Input: part model. Units: mm. Frame: model coordinates. Face numbers are marked on the shaded views. Coordinates: 2 decimals unless noted, no trailing zeros. Loops run counter-clockwise (first coordinate to the right, second up) from the corner with the lowest first, then second, coordinate; pieces in that order, holes last. Notation, with made-up numbers: (85, -27) -> (137, -27) arc R19 ccw to (137, 2) -> close; hole circle Ø1 at (69.5, 51.25). An arc over 180 degrees is marked (long way). Put each result on its own line as item: value. Start each with the question number.
1) Cut plane C-C (y = 18.5). Return the cut outline in (x, z), plus the area to 3 significant figures.
2) Pull-direction query (X, two-part tool) for the marked faces 1, 2, 3 and 4; classes: pulls with the +X half, pulls with the -X half, needs draft (parallel to the pull), parting line crosses it, or undercut.
3) Cut plane A-A (z = 0). Return the cut outline in (x, y), plus the area to 3 significant figures.
4) Material intervals for L1, parallel to X at y = 16, z = -14; L2, parallel to X at y = 15.75, z = 0; L3, parallel to X at y = 3.5, z = 11, sorted ascending.
5) Cut plane B-B (x = 0). Return the cut outline in (y, z).
6) Contact query for flat-ended pins moving along their axis: P1, Ø1.5, axis at x = -18.5, y = 4, coming from the -Z side; P2, Ø6, axis at x = -8, y = 13.5, coming from the -Z side; P3, Ø1.5, axis at x = 1.5, y = 8, coming from the -Z side. Output: stop coordinate, or through.
7) Cut plane D-D (x = -14). Return the cut outline in (y, z), plus the area to 3 significant figures.
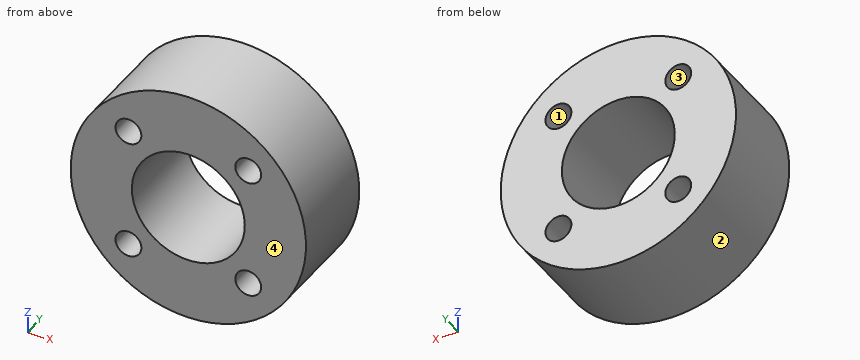
from build123d import *

# Parameters (mm, degrees)
SKETCH_1_R          = 25
EXTRUDE_1_DEPTH     = 20
SKETCH_2_R          = 12
CUT_EXTRUDE_1_DEPTH = 41.620192023
HOLE_WIZARD_M5_1_D  = 5.5


with BuildPart() as part:
    # ｽｹｯﾁ1 → ﾎﾞｽ - 押し出し1 (new body)
    with BuildSketch(Plane(origin=(0, 0, 0), x_dir=(1, 0, 0), z_dir=(0, 1, 0))):
        with Locations(Location((0, 0, 0), (0, 0, 270))):
            Circle(SKETCH_1_R)
    extrude(amount=EXTRUDE_1_DEPTH)

    # ｽｹｯﾁ2 → ｶｯﾄ - 押し出し1 (cut, through all)
    with BuildSketch(Plane(origin=(0, 20, 0), x_dir=(1, 0, 0), z_dir=(0, 1, 0))):
        with Locations(Location((0, 0, 0), (0, 0, 270))):
            Circle(SKETCH_2_R)
    extrude(amount=-CUT_EXTRUDE_1_DEPTH, mode=Mode.SUBTRACT)

    # M5 すきま穴1 (through all)
    with Locations(Plane.XZ):
        with Locations((-12.727922061, 12.727922061), (12.727922061, -12.727922061), (-12.727922061, -12.727922061), (12.727922061, 12.727922061)):
            Hole(HOLE_WIZARD_M5_1_D / 2)


solid = part.part
Results found:
1. outline: circle Ø50 at (0, 0); hole circle Ø5.5 at (-12.73, -12.73); hole circle Ø5.5 at (-12.73, 12.73); hole circle Ø24 at (0, 0); hole circle Ø5.5 at (12.73, -12.73); hole circle Ø5.5 at (12.73, 12.73)
1. area: 1,420 mm2
2. face 1: undercut
2. face 2: parting line crosses it
2. face 3: undercut
2. face 4: needs draft
3. outline: (-25, 0) -> (-12, 0) -> (-12, 20) -> (-25, 20) -> close; (12, 0) -> (25, 0) -> (25, 20) -> (12, 20) -> close
3. area: 520 mm2
4. L1: x = -20.71 to -15.17, -10.29 to 10.29, 15.17 to 20.71
4. L2: x = -25 to -12, 12 to 25
4. L3: x = -22.45 to -14.87, -10.59 to -4.8, 4.8 to 10.59, 14.87 to 22.45
5. outline: (0, -25) -> (20, -25) -> (20, -12) -> (0, -12) -> close; (0, 12) -> (20, 12) -> (20, 25) -> (0, 25) -> close
6. P1: stops at z = -17.61
6. P2: stops at z = -24.49
6. P3: stops at z = -24.99
7. outline: (0, -20.71) -> (20, -20.71) -> (20, -15.17) -> (0, -15.17) -> close; (0, -10.29) -> (20, -10.29) -> (20, 10.29) -> (0, 10.29) -> close; (0, 15.17) -> (20, 15.17) -> (20, 20.71) -> (0, 20.71) -> close
7. area: 633 mm2
